Check sheet for the drawn part. Datum: minimum x, y, z corner. Units: mm. A direction names the side the tool comes from. Coordinates: 2 decimals unless noted, no trailing zeros. Return JSON: item names as keys, results as strings. Group by question number.
Item 1: Scan lines: probe 1 along Z at (x, y) = (1.75, 5.25); probe 2 along Z at (x, y) = (3, 4.25); probe 3 along X at (y, z) = (5.75, 9.5) (1 decimal). Record each from-to range of solid material in increasing order.
Item 2: Tool access check on the marked faces 4, 5 and 6. Record the directions out of +Z, -Z, +X, -X, +Y, -Y that give a thin tool (end or side, any length) a straight path to the whole face; none if there is none.
Item 3: Gauge pin test, flat ends, axial feed: pin 1 (0.8 mm diameter, centred on y = 3.5, z = 9.5, fed in from -X) (3 decimals); pin 2 (1 mm diameter, centred on x = 1, y = 4.5, fed in from -Z); pin 3 (0.8 mm diameter, centred on y = 3.5, z = 9.5, fed in from +X) (3 decimals). Record the tip position at first contact, or that the pin passes through.
Item 4: Draft check along X on the marked faces 1, 2 and 3. Enter one of: pulls with the +X half, pulls with the -X half, needs draft (parallel to the pull), parting line crosses it, or undercut.
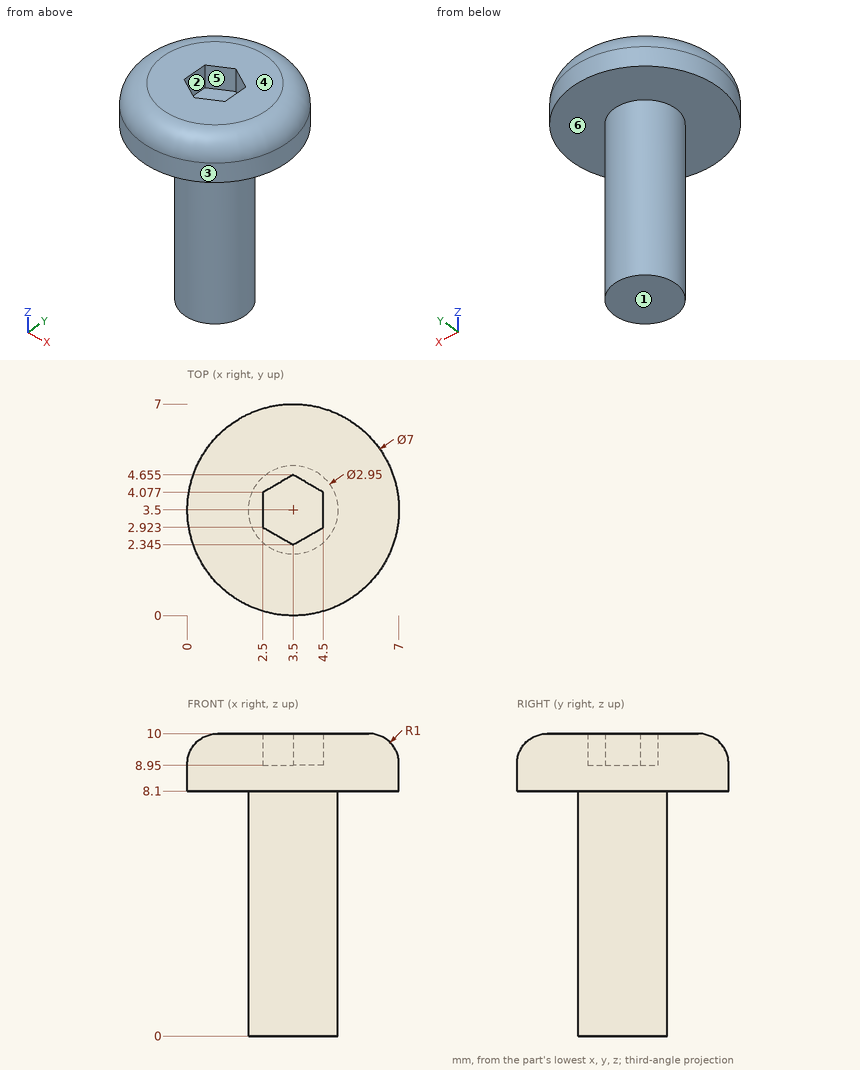
Computed:
{
 "1": {"probe 1": "z = 8.1 to 10", "probe 2": "z = 0 to 8.95", "probe 3": "x = 1 to 6"},
 "2": {"face 4": "+Z, +X, -X, +Y, -Y", "face 5": "+Z", "face 6": "-Z"},
 "3": {"pin 1": "stops at x = 0.005", "pin 2": "stops at z = 8.1", "pin 3": "stops at x = 6.995"},
 "4": {"face 1": "needs draft", "face 2": "undercut", "face 3": "parting line crosses it"}
}
